Verification items for the finished model (mm, model axes). A direction names the side the tool comes from. Round coordinates to 2 decimals unless told otherwise and drop trailing zeros. Order: outer loops, then holes, each group sorted by start corner. A loop starts at its lowest first (then second) coordinate and runs counter-clockwise, first axis right, second up. Notation, with made-up numbers: (77, -19.5) -> (96, -19.5) arc R34 cw to (96, 19.5) -> close; hole circle Ø11 at (52.25, -36). An arc over 180 degrees is marked (long way). Return JSON: item names as keys, results as strings. Group by question number.
Item 1: Sectioned sample at C-C on x = 5.5. Record the cut outline in (y, z), plus the area to 3 significant figures.
Item 2: Draft check along Z on faces 1 (the flat face through (19, -10, 29)), 2 (the flat face through (10, -10, 0)), 3 (the flat face through (1, -9.9, 13.5)). Enter one of: pulls with the +Z half, pulls with the -Z half, needs draft (parallel to the pull), parting line crosses it, or undercut.
Item 3: Sectioned sample at B-B on y = -3.5. Record the cut outline in (x, z).
Item 4: Sectioned sample at D-D on x = 10.5. Record the cut outline in (y, z), plus the area to 3 significant figures.
Item 5: Sectioned sample at A-A on x = 17.25. Record the cut outline in (y, z), plus the area to 3 significant figures.
Item 6: Access from +Z, -Z, +X, -X, +Y, -Y to the whole of each face (thin tool, end or side, straight path). Record for faces 4 (the flat face through (0, -10, 5)), 5 (the flat face through (14, -10, 6)), 6 (the flat face through (6, -9.9, 18.5)).
Item 7: Scan lines: probe 1 along Z at (x, y) = (10.75, -14); probe 2 along Z at (x, y) = (13.5, -9.5); probe 3 along X at (y, z) = (-15.25, 7.25). Record each from-to range of solid material in increasing order. Write a range as from..to.
Item 8: Depth check by flat-ended pin: pin 1 Ø1.8 at (y, z) = (-9, 9) entering from -X. Enter the tip coordinate at first touch or a pass-through.
```python
from build123d import *

# Parameters (mm, degrees)
F1_DEPTH = 20
F2_SIZE  = 2
F3_SIZE  = 2


with BuildPart() as f1:
    # F0 (on Front) → F1 (new body)
    with BuildSketch(Plane.XZ):
        Polygon((0, 7.5), (0, 0), (20, 0), (20, 17.5), (5, 17.5), (5, 25), (15, 25), (15, 22.5), (20, 22.5), (20, 30), (0, 30), (0, 12.5), (15, 12.5), (15, 5), (5, 5), (5, 7.5), align=None)
    extrude(amount=F1_DEPTH)

    # F2
    f2_edges = [f1.edges().sort_by_distance(p)[0] for p in [
        (20, -10, 30),
        (0, -10, 30),
        (0, -10, 12.5),
        (20, -10, 17.5),
        (0, -10, 0),
        (20, -10, 0),
    ]]
    chamfer(f2_edges, length=F2_SIZE)

    # F3
    f3_edges = [f1.edges().sort_by_distance(p)[0] for p in [
        (5, -10, 17.5),
        (5, -10, 5),
        (5, -10, 25),
        (15, -10, 12.5),
        (15, -10, 25),
        (15, -10, 5),
    ]]
    chamfer(f3_edges, length=F3_SIZE)


solid = f1.part
```
Recorded:
{
 "1": {"outline": "(-20, 0) -> (0, 0) -> (0, 6.5) -> (-20, 6.5) -> close; (-20, 12.5) -> (0, 12.5) -> (0, 19) -> (-20, 19) -> close; (-20, 23.5) -> (0, 23.5) -> (0, 30) -> (-20, 30) -> close", "area": "390 mm²"},
 "2": {"face 1": "pulls with the +Z half", "face 2": "pulls with the -Z half", "face 3": "undercut"},
 "3": {"outline": "(0, 2) -> (2, 0) -> (18, 0) -> (20, 2) -> (20, 15.5) -> (18, 17.5) -> (7, 17.5) -> (5, 19.5) -> (5, 23) -> (7, 25) -> (13, 25) -> (15, 23) -> (15, 22.5) -> (20, 22.5) -> (20, 28) -> (18, 30) -> (2, 30) -> (0, 28) -> (0, 14.5) -> (2, 12.5) -> (13, 12.5) -> (15, 10.5) -> (15, 7) -> (13, 5) -> (7, 5) -> (5, 7) -> (5, 7.5) -> (0, 7.5) -> close"},
 "4": {"outline": "(-20, 0) -> (0, 0) -> (0, 5) -> (-20, 5) -> close; (-20, 12.5) -> (0, 12.5) -> (0, 17.5) -> (-20, 17.5) -> close; (-20, 25) -> (0, 25) -> (0, 30) -> (-20, 30) -> close", "area": "300 mm²"},
 "5": {"outline": "(-20, 0) -> (0, 0) -> (0, 17.5) -> (-20, 17.5) -> close; (-20, 22.5) -> (0, 22.5) -> (0, 30) -> (-20, 30) -> close", "area": "500 mm²"},
 "6": {"face 4": "+Z, -Z, -X, +Y, -Y", "face 5": "+Y, -Y", "face 6": "+X, +Y, -Y"},
 "7": {"probe 1": "0..5, 12.5..17.5, 25..30", "probe 2": "0..5.5, 12..17.5, 24.5..30", "probe 3": "0..5, 15..20"},
 "8": {"pin 1": "x = 15"}
}
